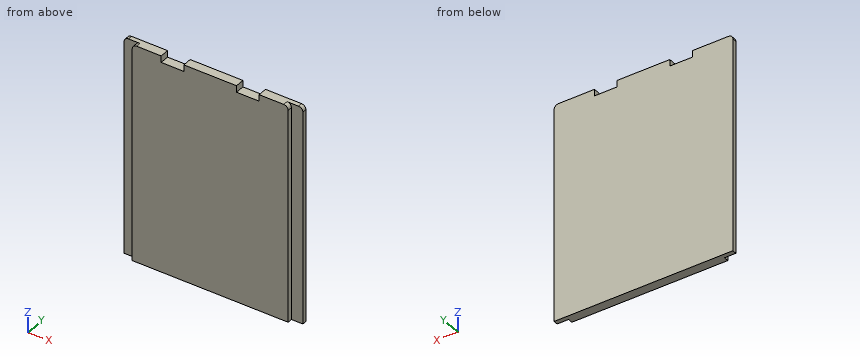
```python
from build123d import *

# Parameters (mm, degrees)
BOSS_EXTRUDE1_DEPTH = 99.6
FILLET1_R           = 2
SKETCH3_W           = 10.297809691
SKETCH3_H           = 3
CUT_EXTRUDE1_DEPTH  = 5
FILLET2_R           = 2


with BuildPart() as part:
    # Sketch2 → Boss-Extrude1 (new body)
    with BuildSketch(Plane.XY):
        Polygon((35.5, 0), (-35.5, 0), (-35.5, 2.2), (-40.7, 2.2), (-40.7, 4.2), (40.7, 4.2), (40.7, 2.2), (35.5, 2.2), align=None)
    extrude(amount=BOSS_EXTRUDE1_DEPTH)

    # Fillet1
    fillet1_edges = [part.edges().sort_by_distance(p)[0] for p in [
        (40.7, 3.2, 99.6),
        (-40.7, 3.2, 99.6),
    ]]
    fillet(fillet1_edges, radius=FILLET1_R)

    # Sketch3 → Cut-Extrude1 (cut)
    with BuildSketch(Plane(origin=(0, 0, 0), x_dir=(-1, 0, 0), z_dir=(0, -1, 0))):
        with Locations((17.151095155, -98.1)):
            Rectangle(SKETCH3_W, SKETCH3_H)
        with Locations((-17.151095155, -98.1)):
            Rectangle(SKETCH3_W, SKETCH3_H)
    extrude(amount=-CUT_EXTRUDE1_DEPTH, mode=Mode.SUBTRACT)

    # Fillet2
    fillet2_edges = [part.edges().sort_by_distance(p)[0] for p in [
        (35.5, 1.1, 99.6),
        (-35.5, 1.1, 99.6),
    ]]
    fillet(fillet2_edges, radius=FILLET2_R)


solid = part.part
```
Model file for the job. Use its own axes, mm. Give positions to 0.01 mm unless a question says otherwise; leave off trailing zeros. Write each loop counter-clockwise with the first axis right and the second up, starting at its lowest first coordinate (ties: lowest second). Pieces come first, ordered by that corner, then holes. Notation, with made-up numbers: (35, -25) - (77, -25) arc R23 ccw to (77, 6) - close; hole circle Ø11 at (-17.75, 50). An arc over 180 degrees is marked (long way). One line per question, with ' | ' between items. Start each with the question number.
(1) Wall check: line 1 along X through (y, z) = (1.6, 6); line 2 along Y through (x, z) = (36, 53); line 3 along Z through (x, y) = (18, 0.3). Give the ranges that are in metal, low to high. Write a range as from..to.
(2) Slice it at C-C on x = 14.5. Write the cut outline in (y, z).
(3) Slice it at B-B on z = 19. Write the cut outline in (x, y).
(4) Slice it at A-A on y = 1.1. Write the cut outline in (x, z), plus the area to 3 significant figures.
(5) Pin check, flat tips, straight feed: P1, Ø2, axis at x = -17, y = 1, coming from the +Z side; P2, Ø1.5, axis at y = 1.5, z = 98, coming from the -X side; P3, Ø0.9, axis at y = 1.5, z = 98.5, coming from the +X side. Stop position of each tip, or through.
Results below:
1) line 1: -35.5..35.5 | line 2: 2.2..4.2 | line 3: 0..96.6
2) outline: (0, 0) - (4.2, 0) - (4.2, 96.6) - (0, 96.6) - close
3) outline: (-40.7, 2.2) - (-35.5, 2.2) - (-35.5, 0) - (35.5, 0) - (35.5, 2.2) - (40.7, 2.2) - (40.7, 4.2) - (-40.7, 4.2) - close
4) outline: (-35.5, 0) - (35.5, 0) - (35.5, 97.6) arc R2 ccw to (33.5, 99.6) - (22.3, 99.6) - (22.3, 96.6) - (12, 96.6) - (12, 99.6) - (-12, 99.6) - (-12, 96.6) - (-22.3, 96.6) - (-22.3, 99.6) - (-33.5, 99.6) arc R2 ccw to (-35.5, 97.6) - close | area: 7,010 mm^2
5) P1: z = 96.6 | P2: x = -40.7 | P3: x = 35.45
